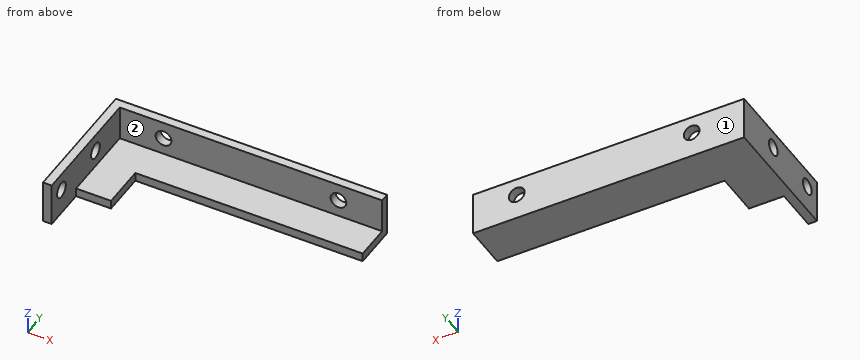
from build123d import *

# Parameters (mm, degrees)
BOSS_EXTRU_1_DEPTH      = 5
ENL_V_MAT_EXTRU_1_DEPTH = 4
ESQUISSE3_R             = 0.9
ENL_V_MAT_EXTRU_2_DEPTH = 10
ESQUISSE4_R             = 0.9
ENL_V_MAT_EXTRU_3_DEPTH = 10


with BuildPart() as part:
    # Esquisse1 → Boss.-Extru.1 (new body)
    with BuildSketch(Plane.XY):
        Polygon((0, 0), (31, 0), (31, -5), (5, -5), (5, -10), (1, -10), (1, -15), (0, -15), align=None)
    extrude(amount=BOSS_EXTRU_1_DEPTH)

    # Esquisse2 → Enlèv. mat.-Extru.1 (cut)
    with BuildSketch(Plane.XY.offset(5)):
        Polygon((1, -10), (1, -1), (31, -1), (31, -5), (5, -5), (5, -10), align=None)
    extrude(amount=-ENL_V_MAT_EXTRU_1_DEPTH, mode=Mode.SUBTRACT)

    # Esquisse3 → Enlèv. mat.-Extru.2 (cut)
    with BuildSketch(Plane(origin=(1, 0, 0), x_dir=(0, 0, -1), z_dir=(1, 0, 0))):
        with Locations((-3, -6)):
            Circle(ESQUISSE3_R)
        with Locations((-3, -13)):
            Circle(ESQUISSE3_R)
    extrude(amount=-ENL_V_MAT_EXTRU_2_DEPTH, mode=Mode.SUBTRACT)

    # Esquisse4 → Enlèv. mat.-Extru.3 (cut)
    with BuildSketch(Plane.XZ.offset(1)):
        with Locations(Location((6, 3, 0), (0, 0, 270))):
            Circle(ESQUISSE4_R)
        with Locations(Location((26, 3, 0), (0, 0, 270))):
            Circle(ESQUISSE4_R)
    extrude(amount=-ENL_V_MAT_EXTRU_3_DEPTH, mode=Mode.SUBTRACT)


solid = part.part
Design review of the part built by this model. Coordinates are the model's own, in mm. Face numbers are marked on the shaded views. A direction names the side the tool comes from. Round coordinates to 2 decimals unless told otherwise and drop trailing zeros. Write each loop counter-clockwise with the first axis right and the second up, starting at its lowest first coordinate (ties: lowest second). Pieces come first, ordered by that corner, then holes. Notation, with made-up numbers: (-13.75, 68) -> (7.25, 68) arc R29 ccw to (7.25, 88) -> close; hole circle Ø9 at (72, -21). An arc over 180 degrees is marked (long way). One line per item, written item: value. Start each with the question number.
Q1. Add section B-B (z = 3). Give the boundary of the cut face in (x, y).
Q2. Add section C-C (y = -13). Give the boundary of the cut face in (x, z), then the cut area to 3 significant figures.
Q3. To check wall thickness, follow probe 1 along Y at (x, z) = (0.2, 3); probe 2 along X at (y, z) = (-0.7, 3); probe 3 along X at (y, z) = (-2, 2.2). State the ranges of each line that lie inside material, in increasing order.
Q4. Tool access review of the marked faces 1 and 2: name each direction out of +Z, -Z, +X, -X, +Y, -Y from which nothing blocks a thin tool from reaching the whole face with its end or side.
Q5. Add section A-A (x = 26). Give the boundary of the cut face in (y, z), then the cut area to 3 significant figures.
Q6. Add section D-D (x = 4). Give the boundary of the cut face in (y, z), then the cut area to 3 significant figures.
Q7. Insertion check: P1, Ø0.5, axis at y = -6.5, z = 0.5, coming from the +X side; P2, Ø2, axis at x = 12.5, z = 3.5, coming from the -Y side; P3, Ø1.1, axis at x = 4, z = 0.5, coming from the -Y side. Each pin has a flat end and moves straight along its axis. Give the tip position at first contact, or say it passes through.
Response:
1. outline: (0, -15) -> (1, -15) -> (1, -13.9) -> (0, -13.9) -> close; (0, -12.1) -> (1, -12.1) -> (1, -6.9) -> (0, -6.9) -> close; (0, -5.1) -> (1, -5.1) -> (1, -1) -> (5.1, -1) -> (5.1, 0) -> (0, 0) -> close; (6.9, -1) -> (25.1, -1) -> (25.1, 0) -> (6.9, 0) -> close; (26.9, -1) -> (31, -1) -> (31, 0) -> (26.9, 0) -> close
2. outline: (0, 0) -> (1, 0) -> (1, 2.1) -> (0, 2.1) -> close; (0, 3.9) -> (1, 3.9) -> (1, 5) -> (0, 5) -> close
2. area: 3.20 mm^2
3. probe 1: y = -15 to -13.9, -12.1 to -6.9, -5.1 to 0
3. probe 2: x = 0 to 5.1, 6.9 to 25.1, 26.9 to 31
3. probe 3: x = 0 to 1
4. face 1: +Z, -Z, +X, -X, +Y
4. face 2: +Z, +X, -Y
5. outline: (-5, 0) -> (0, 0) -> (0, 2.1) -> (-1, 2.1) -> (-1, 1) -> (-5, 1) -> close; (-1, 3.9) -> (0, 3.9) -> (0, 5) -> (-1, 5) -> close
5. area: 7.20 mm^2
6. outline: (-10, 0) -> (0, 0) -> (0, 5) -> (-1, 5) -> (-1, 1) -> (-10, 1) -> close
6. area: 14.0 mm^2
7. P1: stops at x = 5
7. P2: stops at y = -1
7. P3: stops at y = -10
